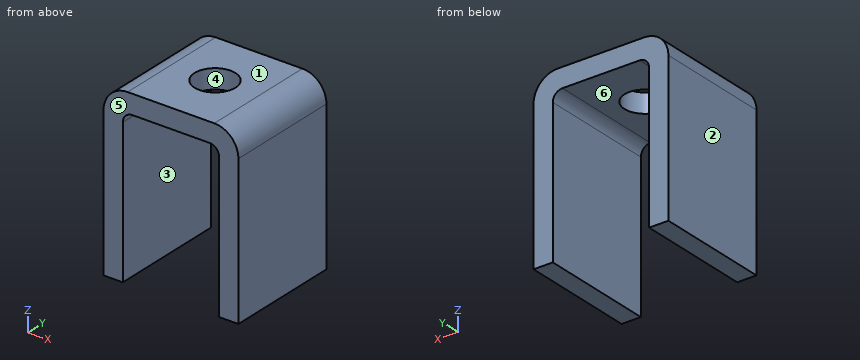
```python
from build123d import *

# Parameters (mm, degrees)
F1_DEPTH = 38.1
F2_R     = 6.35
F3_R     = 15.875
F4_R     = 13.49375
F5_DEPTH = 57.151


with BuildPart() as f1:
    # F0 (on Front) → F1 (new body, symmetric)
    with BuildSketch(Plane.XZ):
        Polygon((31.75, -57.15), (44.45, -57.15), (44.45, 57.15), (-44.45, 57.15), (-44.45, -57.15), (-31.75, -57.15), (-31.75, 44.45), (31.75, 44.45), align=None)
    extrude(amount=F1_DEPTH, both=True)

    # F2
    f2_edges = [f1.edges().sort_by_distance(p)[0] for p in [
        (-31.75, 0, 44.45),
        (31.75, 0, 44.45),
    ]]
    fillet(f2_edges, radius=F2_R)

    # F3
    f3_edges = [f1.edges().sort_by_distance(p)[0] for p in [
        (-44.45, 0, 57.15),
        (44.45, 0, 57.15),
    ]]
    fillet(f3_edges, radius=F3_R)

    # F4 (on Top) → F5 (cut, through all)
    with BuildSketch(Plane.XY):
        Circle(F4_R)
    extrude(amount=F5_DEPTH, mode=Mode.SUBTRACT)


solid = f1.part
```
CAD build for the part. Positions are in the model's coordinates, mm. Face numbers are marked on the shaded views. A direction names the side the tool comes from. Round coordinates to 2 decimals unless told otherwise and drop trailing zeros. Order: outer loops, then holes, each group sorted by start corner. A loop starts at its lowest first (then second) coordinate and runs counter-clockwise, first axis right, second up. Notation, with made-up numbers: (66, 39) - (70, 39) arc R26 ccw to (70, 64) - close; hole circle Ø9 at (21.5, -38). An arc over 180 degrees is marked (long way). Answer in a Markdown table with one row per item. Add a question column.
(1) Band-saw the part on B-B on z = -46. List the corners of the cut face in (x, y).
(2) Band-saw the part on D-D on x = 16.5. List the corners of the cut face in (y, z), and give its area (3 significant figures).
(3) Drop flat-ended pins along their axis: pin 1 Ø6 at (x, y) = (-26, -18) entering from -Z; pin 2 Ø10 at (x, y) = (20, 23.5) entering from -Z; pin 3 Ø1.5 at (x, y) = (25.5, -24) entering from -Z; pin 4 Ø24.5 at (x, y) = (0, 0) entering from -Z. Give the stop position or say it passes through.
(4) Band-saw the part on C-C on y = 0. List the corners of the cut face in (x, z) (3 decimals), and give its area (3 significant figures).
(5) Band-saw the part on A-A on x = 0. List the corners of the cut face in (y, z), and give its area (3 significant figures).
(6) 3-axis set-ups, long thin cutter, end or side, ignore diameter. For the marked faces 5 and 6: which of +Z, -Z, +X, -X, +Y, -Y reach the whole face in a straight line?
(7) Mould opens along X. For the marked faces 1, 2, 3 and 4 say: +X half, -X half, draft (parallel to the pull), parting line (faces both ways), or undercut.
(8) Probe L1, parallel to X at y = 29.5, z = 28; L2, parallel to Y at x = 0, z = 51; L3, parallel to Z at x = -22.5, y = -7. List the from-to ranges inside material, lowest first. Write a range as [from, to].
Data:
| question | item | result |
|---|---|---|
| 1 | outline | (-44.45, -38.1) - (-31.75, -38.1) - (-31.75, 38.1) - (-44.45, 38.1) - close; (31.75, -38.1) - (44.45, -38.1) - (44.45, 38.1) - (31.75, 38.1) - close |
| 2 | outline | (-38.1, 44.45) - (38.1, 44.45) - (38.1, 57.15) - (-38.1, 57.15) - close |
| 2 | area | 968 mm^2 |
| 3 | pin 1 | stops at z = 43.33 |
| 3 | pin 2 | stops at z = 44.45 |
| 3 | pin 3 | stops at z = 44.39 |
| 3 | pin 4 | passes through |
| 4 | outline | (-44.45, -57.15) - (-31.75, -57.15) - (-31.75, 38.1) arc R6.35 cw to (-25.4, 44.45) - (-13.494, 44.45) - (-13.494, 57.15) - (-28.575, 57.15) arc R15.875 ccw to (-44.45, 41.275) - close; (13.494, 44.45) - (25.4, 44.45) arc R6.35 cw to (31.75, 38.1) - (31.75, -57.15) - (44.45, -57.15) - (44.45, 41.275) arc R15.875 ccw to (28.575, 57.15) - (13.494, 57.15) - close |
| 4 | area | 3,280 mm^2 |
| 5 | outline | (-38.1, 44.45) - (-13.49, 44.45) - (-13.49, 57.15) - (-38.1, 57.15) - close; (13.49, 44.45) - (38.1, 44.45) - (38.1, 57.15) - (13.49, 57.15) - close |
| 5 | area | 625 mm^2 |
| 6 | face 5 | +Z, -Z, +X, -X, -Y |
| 6 | face 6 | -Z, +Y, -Y |
| 7 | face 1 | draft |
| 7 | face 2 | -X half |
| 7 | face 3 | undercut |
| 7 | face 4 | undercut |
| 8 | L1 | x = [-44.45, -31.75], [31.75, 44.45] |
| 8 | L2 | y = [-38.1, -13.49], [13.49, 38.1] |
| 8 | L3 | z = [44.45, 57.15] |
